Part model, mm, in its own coordinate system. A direction names the side the tool comes from. Give positions to 0.01 mm unless a question says otherwise; leave off trailing zeros. Order: outer loops, then holes, each group sorted by start corner. A loop starts at its lowest first (then second) coordinate and runs counter-clockwise, first axis right, second up. Notation, with made-up numbers: (76.5, -32.75) - (80.5, -32.75) arc R28 ccw to (80.5, 4.25) - close; hole circle Ø3 at (16.25, 20.25). An arc over 180 degrees is marked (long way). Use one line per item in the form item = value. Start each with the question number.
1. Pin check, flat tips, straight feed: P1, Ø10, axis at y = 31, z = -0.5, coming from the -X side; P2, Ø8, axis at x = 54.5, y = 55.5, coming from the -Z side; P3, Ø19, axis at x = 0, z = 60, coming from the -Y side. Stop position of each tip, or through.
2. Band-saw the part on B-B, the plane x = 0. List the corners of the cut face in (y, z).
3. Pull direction Z, two halves, no side cores. Call faces 3 (the face through (-34.608, 52.22, 66.538)), 4 (the face through (-1, 62.36, -18)), 5 (the face through (1.301, 52.5, 65.857)): +Z half, -Z half, draft (parallel to the pull), parting line (faces both ways), or undercut.
4. Drill centre lines: line 1 (Z direction, x = 0, y = 52.5); line 2 (X direction, y = 54, z = -5); line 3 (Y direction, x = -54, z = -22). Where is each one in solid material? Low to high.
5. Band-saw the part on D-D, the plane z = 0. List the corners of the cut face in (x, y).
6. Band-saw the part on C-C, the plane x = -60. List the corners of the cut face in (y, z).
7. Band-saw the part on A-A, the plane z = 60. List the corners of the cut face in (x, y), plus the area to 3 significant figures.
8. Tool access for faces 1 (the face through (4.42, 52.5, -64.06)), 2 (the face through (-47.69, 29.68, -15.02)): list every direction of +Z, -Z, +X, -X, +Y, -Y with a clear straight run to the whole face (end or side of a thin tool).
from build123d import *

# Parameters (mm, degrees)
CORTAR_EXTRUIR1_DEPTH      = 112.691539518
CORTAR_EXTRUIR1_DEPTH_BACK = 29
CROQUIS4_R                 = 6
REDONDEO3_R                = 10


with BuildPart() as part:
    # Croquis1 → Revolución1 (revolve)
    with BuildSketch(Plane.XY, mode=Mode.PRIVATE) as revoluci_n1_sk:
        Polygon((75, 42.359797144), (50, 42.359797144), (50, 7.359797144), (17.5, 7.359797144), (17.5, 42.359797144), (17.5, 62.359797144), (75, 62.359797144), align=None)
    revolve(revoluci_n1_sk.sketch.rotate(Axis((0, 71.893155669, 0), (0, -1, 0)), 180), axis=Axis((0, 71.893155669, 0), (0, -1, 0)))

    # Croquis4 → Cortar-Extruir1 (cut, two sides: drawn at the far end of the back side and taken through both)
    with BuildSketch(Plane.XZ.offset(-42.359797144).offset(-CORTAR_EXTRUIR1_DEPTH_BACK)):
        with Locations(Location((0, 60, 0), (0, 0, 180))):
            Circle(CROQUIS4_R)
        with Locations(Location((60, 0, 0), (0, 0, 180))):
            Circle(CROQUIS4_R)
        with Locations(Location((0, -60, 0), (0, 0, 180))):
            Circle(CROQUIS4_R)
        with Locations(Location((-60, 0, 0), (0, 0, 180))):
            Circle(CROQUIS4_R)
    extrude(amount=CORTAR_EXTRUIR1_DEPTH + CORTAR_EXTRUIR1_DEPTH_BACK, mode=Mode.SUBTRACT)

    # Redondeo3
    redondeo3_edges = [part.edges().sort_by_distance(p)[0] for p in [
        (17.5, 7.359797144, 0),
        (50, 7.359797144, 0),
    ]]
    fillet(redondeo3_edges, radius=REDONDEO3_R)


solid = part.part
From the geometry:
q1.P1 = -50
q1.P2 = -55.45
q1.P3 = 42.36
q2.outline = (7.36, -40) arc R10 ccw to (17.36, -50) - (42.36, -50) - (42.36, -54) - (62.36, -54) - (62.36, -17.5) - (17.36, -17.5) arc R10 ccw to (7.36, -27.5) - close; (7.36, 27.5) arc R10 ccw to (17.36, 17.5) - (62.36, 17.5) - (62.36, 54) - (42.36, 54) - (42.36, 50) - (17.36, 50) arc R10 ccw to (7.36, 40) - close; (42.36, -75) - (62.36, -75) - (62.36, -66) - (42.36, -66) - close; (42.36, 66) - (62.36, 66) - (62.36, 75) - (42.36, 75) - close
q3.face_3 = parting line
q3.face_4 = draft
q3.face_5 = undercut
q4.line_1 = -75 to -66, -54 to -17.5, 17.5 to 54, 66 to 75
q4.line_2 = -74.83 to -63.32, -56.68 to -16.77, 16.77 to 56.68, 63.32 to 74.83
q4.line_3 = 42.36 to 62.36
q5.outline = (-75, 42.36) - (-66, 42.36) - (-66, 62.36) - (-75, 62.36) - close; (-54, 42.36) - (-50, 42.36) - (-50, 17.36) arc R10 ccw to (-40, 7.36) - (-27.5, 7.36) arc R10 ccw to (-17.5, 17.36) - (-17.5, 62.36) - (-54, 62.36) - close; (17.5, 17.36) arc R10 ccw to (27.5, 7.36) - (40, 7.36) arc R10 ccw to (50, 17.36) - (50, 42.36) - (54, 42.36) - (54, 62.36) - (17.5, 62.36) - close; (66, 42.36) - (75, 42.36) - (75, 62.36) - (66, 62.36) - close
q6.outline = (42.36, -45) - (62.36, -45) - (62.36, -6) - (42.36, -6) - close; (42.36, 6) - (62.36, 6) - (62.36, 45) - (42.36, 45) - close
q7.outline = (-45, 42.36) - (-6, 42.36) - (-6, 62.36) - (-45, 62.36) - close; (6, 42.36) - (45, 42.36) - (45, 62.36) - (6, 62.36) - close
q7.area = 1,560 mm²
q8.face_1 = +Y, -Y
q8.face_2 = -Y
